Read the model definition and answer for the solid it produces. Units are mm, in the model's axes. Face numbers are marked on the shaded views. A direction names the side the tool comes from. Coordinates: 2 decimals unless noted, no trailing zeros. Loops run counter-clockwise (first coordinate to the right, second up) from the corner with the lowest first, then second, coordinate; pieces in that order, holes last. Notation, with made-up numbers: M -17,-7 L 34,-7 A7 ccw 34,-2 Z; hole C 10,49.5 d9. An arc over 180 degrees is marked long. One line per item, written item: value. Start each with the question number.
1. Consider probe 1 along Y at (x, z) = (158.5, 30.5); probe 2 along X at (y, z) = (10.5, 2.5); probe 3 along Y at (x, z) = (209.5, 21). Determine where each line is inside the solid, lowest interval first.
2. The part is cut by section A-A (z = 36). Write down the section's boundary in (x, y), then the cut area to 3 significant figures.
3. The part is cut by section B-B (x = 125). Write down the section's boundary in (y, z).
4. Flat-ended cylindrical pins translate along their axes: pin 1 (1.5 mm diameter, centred on x = 202.5, z = 36, fed in from -Y); pin 2 (6 mm diameter, centred on y = 34, z = 22, fed in from +X). Find the tip coordinate at first contact, or state that the pin passes through.
5. For the marked faces 1 and 2, determine the directions among +Z, -Z, +X, -X, +Y, -Y from which every point of the face is accessible in a straight line to the end or side of a thin tool.
6. The part is cut by section C-C (y = 19). Write down the section's boundary in (x, z).
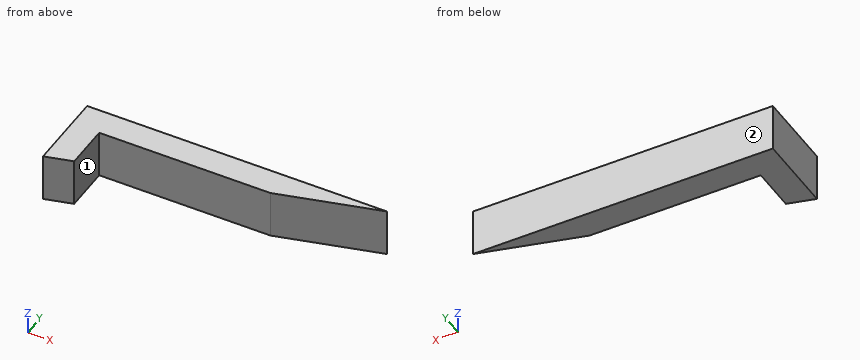
```python
from build123d import *

# Parameters (mm, degrees)
SKETCH1_W           = 25.4
SKETCH1_H           = 25.4
BOSS_EXTRUDE1_DEPTH = 44.958


with BuildPart() as part:
    # Sketch1 → Boss-Extrude1 (new body)
    with BuildSketch(Plane.XY):
        Polygon((-12.7, 0), (12.7, 6.805909488), (12.7, 48.930936062), (-12.7, 48.930936062), align=None)
        with Locations((0, 61.630936062)):
            Rectangle(SKETCH1_W, SKETCH1_H)
        Polygon((12.7, 74.330936062), (12.7, 48.930936062), (172.856591106, 48.930936062), (267.650681618, 74.330936062), align=None)
    extrude(amount=BOSS_EXTRUDE1_DEPTH)


solid = part.part
```
Answer block:
1. probe 1: y = 48.93 to 74.33
1. probe 2: x = -12.7 to 12.7
1. probe 3: y = 58.75 to 74.33
2. outline: M -12.7,0 L 12.7,6.81 L 12.7,48.93 L 172.86,48.93 L 267.65,74.33 L -12.7,74.33 Z
2. area: 7,070 mm2
3. outline: M 48.93,0 L 74.33,0 L 74.33,44.96 L 48.93,44.96 Z
4. pin 1: stops at y = 56.67
4. pin 2: stops at x = 12.7
5. face 1: +Z, -Z, +X, -Y
5. face 2: +Z, -Z, +X, -X, +Y
6. outline: M -12.7,0 L 12.7,0 L 12.7,44.96 L -12.7,44.96 Z
